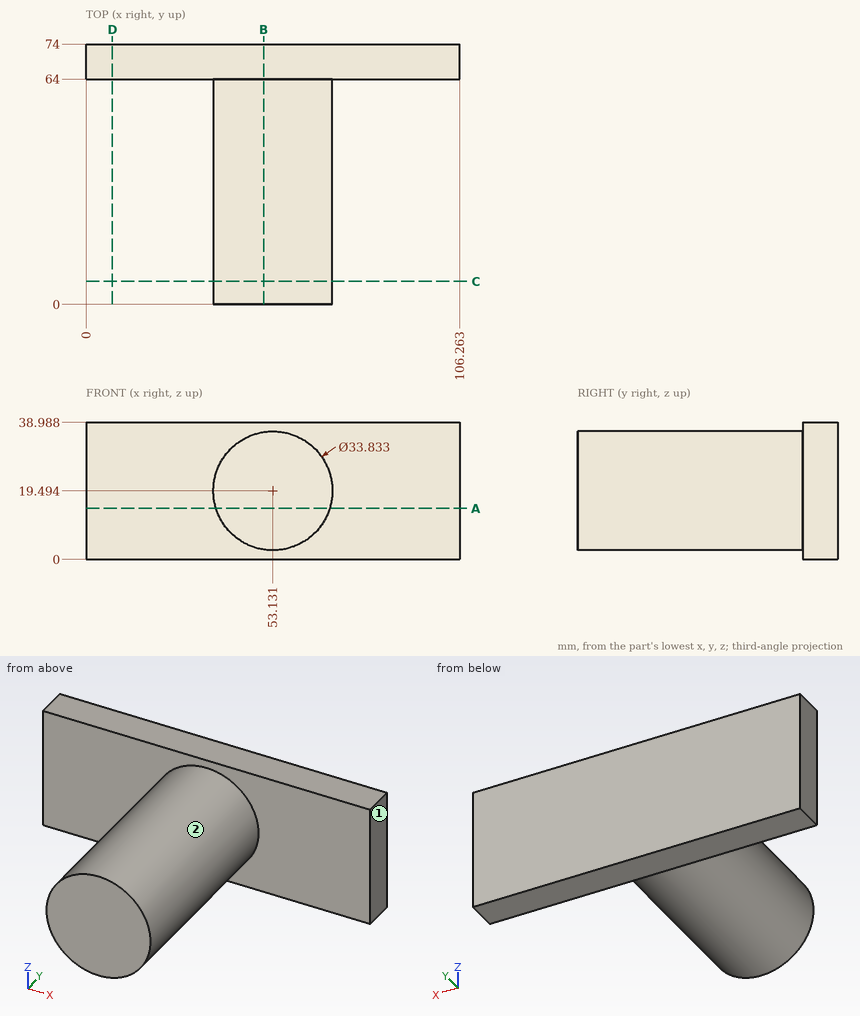
Can you work these out from the drawing? Everything is in mm from the part's minimum corner. A direction names the side the tool comes from. Round coordinates to 2 decimals unless told otherwise and drop trailing zeros. Loops run counter-clockwise (first coordinate to the right, second up) from the corner with the lowest first, then second, coordinate; pieces in that order, holes last. Notation, with made-up numbers: (42, 26) - (97, 26) arc R21 ccw to (97, 43) - close; hole circle Ø11 at (-39.75, 86). An arc over 180 degrees is marked (long way). Write item = value, one per line. Start each with the question number.
(1) If we section it at B-B (x = 50.5): Please give me the cut outline in (y, z) (1 decimal), and give its area (3 significant figures).
(2) For P1, Ø12, axis at x = 14.5, z = 10, coming from the -Y side; P2, Ø4, axis at x = 36.5, y = 49, coming from the -Z side (1 decimal), each with a flat end and sliding along its axis, tell me the tip position at first contact or that it passes through.
(3) If we section it at A-A (z = 14.5): Please give me the cut outline in (x, y) (1 decimal), and give its area (3 significant figures).
(4) For the marked faces 1 and 2, which set-ups out of +Z, -Z, +X, -X, +Y, -Y let a thin tool reach every point of the face, with its end or its side?
(5) If we section it at D-D (x = 7.5): Please give me the cut outline in (y, z).
(6) If we section it at C-C (y = 6.5): Please give me the cut outline in (x, z), and give its area (3 significant figures).
(7) If I drill on probe 1 along Y at (x, z) = (95.5, 11.5); probe 2 along Z at (x, y) = (61, 53.5); probe 3 along X at (y, z) = (47, 25) (1 decimal), over which ranges is the centre line in solid material (lowest first)? Write a range as [from, to].
Ans:
q1.outline = (0, 2.8) - (64, 2.8) - (64, 0) - (74, 0) - (74, 39) - (64, 39) - (64, 36.2) - (0, 36.2) - close
q1.area = 2,530 mm²
q2.P1 = 64
q2.P2 = 11
q3.outline = (0, 64) - (37, 64) - (37, 0) - (69.3, 0) - (69.3, 64) - (106.3, 64) - (106.3, 74) - (0, 74) - close
q3.area = 3,130 mm²
q4.face_1 = +Z, -Z, +X, +Y, -Y
q4.face_2 = -Y
q5.outline = (64, 0) - (74, 0) - (74, 38.99) - (64, 38.99) - close
q6.outline = circle Ø33.83 at (53.13, 19.49)
q6.area = 899 mm²
q7.probe_1 = [64, 74]
q7.probe_2 = [4.52, 34.47]
q7.probe_3 = [37.1, 69.1]
